Geometry: final body of the model. Coordinates: model frame, mm. Give positions to 0.01 mm unless a question says otherwise; leave off trailing zeros. Loops run counter-clockwise (first coordinate to the right, second up) from the corner with the lowest first, then second, coordinate; pieces in that order, holes last.
from build123d import *

# Parameters (mm, degrees)
SKETCH1_W           = 152.4
SKETCH1_H           = 76.2
BOSS_EXTRUDE1_DEPTH = 3.175
CUT_EXTRUDE1_DEPTH  = 3.175
FILLET2_R           = 2.54
FILLET3_R           = 2.54
SKETCH5_R           = 7.62
CUT_EXTRUDE2_DEPTH  = 3.175
SKETCH6_R           = 1.27
CUT_EXTRUDE3_DEPTH  = 3.175
SKETCH7_R           = 1.0033
CUT_EXTRUDE4_DEPTH  = 86.253332046


with BuildPart() as part:
    # Sketch1 → Boss-Extrude1 (new body)
    with BuildSketch(Plane(origin=(0, 0, 0), x_dir=(1, 0, 0), z_dir=(0, 1, 0))):
        Rectangle(SKETCH1_W, SKETCH1_H)
    extrude(amount=BOSS_EXTRUDE1_DEPTH)

    # Sketch4 → Cut-Extrude1 (cut)
    with BuildSketch(Plane(origin=(0, 3.175, 0), x_dir=(1, 0, 0), z_dir=(0, 1, 0))):
        with BuildLine():
            Line((0, 38.1), (76.2, 38.1))
            Line((76.2, 38.1), (76.2, 12.7))
            ThreePointArc((76.2, 12.7), (40.160926284, 31.582778852), (0, 38.1))
        make_face()
        with BuildLine():
            Line((76.2, -38.1), (76.2, -12.7))
            ThreePointArc((76.2, -12.7), (40.160926284, -31.582778852), (0, -38.1))
            Line((0, -38.1), (76.2, -38.1))
        make_face()
    extrude(amount=-CUT_EXTRUDE1_DEPTH, mode=Mode.SUBTRACT)

    # Fillet2
    fillet2_edges = [part.edges().sort_by_distance(p)[0] for p in [
        (76.2, 1.5875, -12.7),
        (76.2, 1.5875, 12.7),
    ]]
    fillet(fillet2_edges, radius=FILLET2_R)

    # Fillet3
    fillet3_edges = [part.edges().sort_by_distance(p)[0] for p in [
        (-76.2, 1.5875, -38.1),
        (-76.2, 1.5875, 38.1),
    ]]
    fillet(fillet3_edges, radius=FILLET3_R)

    # Sketch5 → Cut-Extrude2 (cut)
    with BuildSketch(Plane(origin=(0, 3.175, 0), x_dir=(1, 0, 0), z_dir=(0, 1, 0))):
        with Locations(Location((50.8, 0, 0), (0, 0, 270))):
            Circle(SKETCH5_R)
    extrude(amount=-CUT_EXTRUDE2_DEPTH, mode=Mode.SUBTRACT)

    # Sketch6 → Cut-Extrude3 (cut)
    with BuildSketch(Plane(origin=(0, 3.175, 0), x_dir=(1, 0, 0), z_dir=(0, 1, 0))):
        with Locations(Location((-63.5, 25.4, 0), (0, 0, 270))):
            Circle(SKETCH6_R)
        with Locations(Location((-63.5, -25.4, 0), (0, 0, 270))):
            Circle(SKETCH6_R)
        with Locations(Location((-24.13, 25.4, 0), (0, 0, 270))):
            Circle(SKETCH6_R)
        with Locations(Location((-24.13, -25.4, 0), (0, 0, 270))):
            Circle(SKETCH6_R)
    extrude(amount=-CUT_EXTRUDE3_DEPTH, mode=Mode.SUBTRACT)

    # Sketch7 → Cut-Extrude4 (cut, through all)
    with BuildSketch(Plane(origin=(0, 3.175, 0), x_dir=(1, 0, 0), z_dir=(0, 1, 0))):
        with Locations(Location((70.485, 0, 0), (0, 0, 270))):
            Circle(SKETCH7_R)
        with Locations(Location((31.115, 0, 0), (0, 0, 270))):
            Circle(SKETCH7_R)
    extrude(amount=-CUT_EXTRUDE4_DEPTH, mode=Mode.SUBTRACT)


solid = part.part
Item 1: Section query D-D on x = 28.5. Return loops of the section in (y, z) (3 decimals).
Values follow:
outline: (0, -34.861) - (3.175, -34.861) - (3.175, 34.861) - (0, 34.861) - close
Item 2: Section query C-C on z = -15. Return loops of the section in (x, y) (3 decimals).
Values follow:
outline: (-76.2, 0) - (73.033, 0) - (73.033, 3.175) - (-76.2, 3.175) - close
Item 3: Section query A-A on y = 1.6. Return loops of the section in (x, z) (3 decimals).
Values follow:
outline: (-76.2, -35.56) arc R2.54 ccw to (-73.66, -38.1) - (0, -38.1) arc R127 ccw to (75.163, -13.469) arc R2.54 ccw to (76.2, -11.422) - (76.2, 11.422) arc R2.54 ccw to (75.163, 13.469) arc R127 ccw to (0, 38.1) - (-73.66, 38.1) arc R2.54 ccw to (-76.2, 35.56) - close; hole circle Ø2.54 at (-63.5, -25.4); hole circle Ø2.54 at (-63.5, 25.4); hole circle Ø2.54 at (-24.13, -25.4); hole circle Ø2.54 at (-24.13, 25.4); hole circle Ø2.007 at (31.115, 0); hole circle Ø15.24 at (50.8, 0); hole circle Ø2.007 at (70.485, 0)
Item 4: Ray query, probe 1 along X at (y, z) = (2.4, 0); probe 2 along X at (y, z) = (2.35, -26.5); probe 3 along X at (y, z) = (1.25, 25.4). Return the intervals inside material, ascending.
Values follow:
probe 1: x = -76.2 to 30.11, 32.12 to 43.18, 58.42 to 69.48, 71.49 to 76.2
probe 2: x = -76.2 to -64.13, -62.87 to -24.76, -23.5 to 53.03
probe 3: x = -76.2 to -64.77, -62.23 to -25.4, -22.86 to 55.36
Item 5: Section query B-B on x = 50.8. Return loops of the section in (y, z) (3 decimals).
Values follow:
outline: (0, -27.497) - (3.175, -27.497) - (3.175, -7.62) - (0, -7.62) - close; (0, 7.62) - (3.175, 7.62) - (3.175, 27.497) - (0, 27.497) - close
Item 6: Pin query (flat end, axial travel): pin 1 (2 mm diameter, centred on x = -24.13, z = -25.4, fed in from -Y). Return the tip coordinate at first contact, or that it passes through.
Values follow:
pin 1: passes through
Item 7: Draft query along Z for faces 1 (the face through (40.08, 1.61, 31.61)), 2 (the face through (-37, 2, -38.1)), 3 (the face through (43.36, 1.61, -1.65)). Return one class per face: +Z half, -Z half, draft (parallel to the pull), parting line (faces both ways), or undercut.
Values follow:
face 1: +Z half
face 2: -Z half
face 3: undercut
